Read the model definition and answer for the solid it produces. Units are mm, in the model's axes. A direction names the side the tool comes from. Give positions to 0.01 mm unless a question says otherwise; leave off trailing zeros. Write each loop counter-clockwise with the first axis right and the second up, starting at its lowest first coordinate (ties: lowest second). Pieces come first, ordered by that corner, then holes. Notation, with made-up numbers: (69.5, 23) - (101.5, 23) arc R21 cw to (101.5, 47) - close; hole circle Ø9 at (81, 88.25). An arc over 180 degrees is marked (long way). Answer as CSV lines item,"result".
```python
from build123d import *

# Parameters (mm, degrees)
ESQUISSE1_W                = 143
ESQUISSE1_H                = 16
BOSS_EXTRU_1_DEPTH         = 3
ESQUISSE2_W                = 143
ESQUISSE2_H                = 3
BOSS_EXTRU_2_DEPTH         = 13
ESQUISSE4_R                = 1.5
ENL_V_MAT_EXTRU_1_DEPTH    = 10
R_P_TITION_LIN_AIRE1_COUNT = 9
R_P_TITION_LIN_AIRE1_PITCH = 16
ESQUISSE5_R                = 1.5
ENL_V_MAT_EXTRU_2_DEPTH    = 10
R_P_TITION_LIN_AIRE2_COUNT = 9
R_P_TITION_LIN_AIRE2_PITCH = 16


with BuildPart() as part:
    # Esquisse1 → Boss.-Extru.1 (new body)
    with BuildSketch(Plane.XY):
        with Locations((71.5, 8)):
            Rectangle(ESQUISSE1_W, ESQUISSE1_H)
    extrude(amount=BOSS_EXTRU_1_DEPTH)

    # Esquisse2 → Boss.-Extru.2 (add)
    with BuildSketch(Plane.XY.offset(3)):
        with Locations((71.5, 14.5)):
            Rectangle(ESQUISSE2_W, ESQUISSE2_H)
    extrude(amount=BOSS_EXTRU_2_DEPTH)

    # Esquisse4 → Enlèv. mat.-Extru.1 (cut)
    with BuildSketch(Plane(origin=(0, 0, 0), x_dir=(-1, 0, 0), z_dir=(0, 0, -1))):
        with Locations((-134, 8)):
            Circle(ESQUISSE4_R)
    enl_v_mat_extru_1 = extrude(amount=-ENL_V_MAT_EXTRU_1_DEPTH, mode=Mode.SUBTRACT)

    # Répétition linéaire1: Enlèv. mat.-Extru.1 ×9
    with Locations(*[(-i * R_P_TITION_LIN_AIRE1_PITCH, 0, 0) for i in range(1, R_P_TITION_LIN_AIRE1_COUNT)]):
        add(enl_v_mat_extru_1, mode=Mode.SUBTRACT)

    # Esquisse5 → Enlèv. mat.-Extru.2 (cut)
    with BuildSketch(Plane(origin=(0, 16, 0), x_dir=(1, 0, 0), z_dir=(0, 1, 0))):
        with Locations(Location((134, -8, 0), (0, 0, 270))):
            Circle(ESQUISSE5_R)
    enl_v_mat_extru_2 = extrude(amount=-ENL_V_MAT_EXTRU_2_DEPTH, mode=Mode.SUBTRACT)

    # Répétition linéaire2: Enlèv. mat.-Extru.2 ×9
    with Locations(*[(-i * R_P_TITION_LIN_AIRE2_PITCH, 0, 0) for i in range(1, R_P_TITION_LIN_AIRE2_COUNT)]):
        add(enl_v_mat_extru_2, mode=Mode.SUBTRACT)


solid = part.part
```
(1) Find the intervals of material crossed by L1, parallel to Y at x = 6, z = 1.05; L2, parallel to Y at x = 26, z = 10.25, in increasing order.
Worked out:
L1,"y = 0 to 6.5, 9.5 to 16"
L2,"y = 13 to 16"
(2) Each of these flat-tipped pins is pushed along its axis until it touches: P1, Ø3.5, axis at x = 86, z = 8, coming from the -Y side; P2, Ø2.5, axis at x = 6, y = 8, coming from the +Z side; P3, Ø4, axis at x = 47.5, y = 5.5, coming from the +Z side. Where does it stop, or does it pass through?
Worked out:
P1,"stops at y = 13"
P2,"passes through"
P3,"stops at z = 3"
(3) For faces 1 (the flat face through (70, 13, 11)), 2 (the cylindrical face through (119.5, 8.07, 1.48)), determine the directions among +Z, -Z, +X, -X, +Y, -Y from which every point of the face is accessible in a straight line to the end or side of a thin tool.
Worked out:
face 1,"+Z, +X, -X, -Y"
face 2,"+Z, -Z"
(4) A cutting plane is placed at B-B (y = 14.25). Count the separate pieces of the cut face and the enclosed holes in it, and give its area (3 significant figures).
Worked out:
separate pieces,"1"
enclosed holes,"9"
area,"2,220 mm^2"
(5) The mould has two halves that part along Z. Classify faces 3 (the cylindrical face through (68.614, 7.425, 1.479)), 4 (the cylindrical face through (135.487, 14.521, 7.805)), 5 (the flat face through (70, 15, 16)), 6 (the cylindrical face through (36.536, 14.521, 7.675)): +Z half, -Z half, draft (parallel to the pull), parting line (faces both ways), or undercut.
Worked out:
face 3,"draft"
face 4,"undercut"
face 5,"+Z half"
face 6,"undercut"
(6) A cutting plane is placed at A-A (x = 102). Write down the section's boundary in (y, z).
Worked out:
outline,"(0, 0) - (6.5, 0) - (6.5, 3) - (0, 3) - close; (9.5, 0) - (16, 0) - (16, 6.5) - (13, 6.5) - (13, 3) - (9.5, 3) - close; (13, 9.5) - (16, 9.5) - (16, 16) - (13, 16) - close"
